Could you check a few things on this model? Use its own coordinates, in mm. Coordinates: 2 decimals unless noted, no trailing zeros. Order: outer loops, then holes, each group sorted by start corner. A loop starts at its lowest first (then second) coordinate and runs counter-clockwise, first axis right, second up. Notation, with made-up numbers: M 17.25,46.5 L 51.25,46.5 A29 ccw 51.25,84.5 Z; hole C -22.75,21 d6. An arc over 180 degrees is marked long. Write item = value, one per line. Start each with the question number.
from build123d import *

# Parameters (mm, degrees)
SKETCH2_R           = 1.75
BOSS_EXTRUDE1_DEPTH = 1
BOSS_EXTRUDE3_START = -1
SKETCH4_R           = 1.75
SKETCH4_R_2         = 1.744098306
BOSS_EXTRUDE3_DEPTH = 1


with BuildPart() as part:
    # Sketch2 → Boss-Extrude1 (new body)
    with BuildSketch(Plane.XY):
        with BuildLine():
            Line((0, 3), (0, 27))
            ThreePointArc((0, 27), (-0.878679656, 29.121320344), (-3, 30))
            Line((-3, 30), (-97, 30))
            ThreePointArc((-97, 30), (-99.121320344, 29.121320344), (-100, 27))
            Line((-100, 27), (-100, 3))
            ThreePointArc((-100, 3), (-99.121320344, 0.878679656), (-97, 0))
            Line((-97, 0), (-3, 0))
            ThreePointArc((-3, 0), (-0.878679656, 0.878679656), (0, 3))
        make_face()
        with Locations((-96, 18)):
            Circle(SKETCH2_R, mode=Mode.SUBTRACT)
        with Locations((-4, 18)):
            Circle(SKETCH2_R, mode=Mode.SUBTRACT)
        with BuildLine():
            Line((-97, 27), (-3, 27))
            Line((-3, 27), (-3, 21.872983346))
            ThreePointArc((-3, 21.872983346), (-8, 18), (-3, 14.127016654))
            Line((-3, 14.127016654), (-3, 3))
            Line((-3, 3), (-97, 3))
            Line((-97, 3), (-97, 14.127016654))
            ThreePointArc((-97, 14.127016654), (-92, 18), (-97, 21.872983346))
            Line((-97, 21.872983346), (-97, 27))
        make_face(mode=Mode.SUBTRACT)
    extrude(amount=BOSS_EXTRUDE1_DEPTH)

    # Sketch4 → Boss-Extrude3 (add)
    with BuildSketch(Plane.XY.offset(1).offset(BOSS_EXTRUDE3_START)):
        with BuildLine():
            Line((-97.171540794, 30.25), (-2.828459206, 30.25))
            ThreePointArc((-2.828459206, 30.25), (-0.651659826, 29.348340174), (0.25, 27.171540794))
            Line((0.25, 27.171540794), (0.25, 2.828459206))
            ThreePointArc((0.25, 2.828459206), (-0.651659826, 0.651659826), (-2.828459206, -0.25))
            Line((-2.828459206, -0.25), (-97.171540794, -0.25))
            ThreePointArc((-97.171540794, -0.25), (-99.348340174, 0.651659826), (-100.25, 2.828459206))
            Line((-100.25, 2.828459206), (-100.25, 27.171540794))
            ThreePointArc((-100.25, 27.171540794), (-99.348340174, 29.348340174), (-97.171540794, 30.25))
        make_face()
        with Locations((-96, 18)):
            Circle(SKETCH4_R, mode=Mode.SUBTRACT)
        with Locations((-4, 18)):
            Circle(SKETCH4_R_2, mode=Mode.SUBTRACT)
        with BuildLine():
            Line((-96.75, 26.75), (-3.25, 26.75))
            Line((-3.25, 26.75), (-3.25, 22.183300133))
            ThreePointArc((-3.25, 22.183300133), (-8.25, 18), (-3.25, 13.816699867))
            Line((-3.25, 13.816699867), (-3.25, 3.25))
            Line((-3.25, 3.25), (-96.75, 3.25))
            Line((-96.75, 3.25), (-96.75, 13.816699867))
            ThreePointArc((-96.75, 13.816699867), (-91.75, 18), (-96.75, 22.183300133))
            Line((-96.75, 22.183300133), (-96.75, 26.75))
        make_face(mode=Mode.SUBTRACT)
    extrude(amount=BOSS_EXTRUDE3_DEPTH)


solid = part.part
(1) Imagine slicing it at B-B on y = 18. List the corners of the cut face in (x, z) for me, plus the area to 3 significant figures.
(2) Imagine slicing it at A-A on y = 24. List the corners of the cut face in (x, z) for me, plus the area to 3 significant figures.
(3) Thinking about a two-plate mould opening in Y: for faces 1 (the flat face through (-50, 27, 1)), 2 (the cylindrical face through (-91.75, 17.9, 0.49)), 3 (the cylindrical face through (-0.628, 0.676, 0.493)), which applies, released by +Y, released by -Y, zero draft, split by the parting line, or undercut?
(4) Please list where these lines run through material, in increasing order: probe 1 along Y at (x, z) = (-96, 0.5); probe 2 along Y at (x, z) = (-83.5, 0.15); probe 3 along Y at (x, z) = (-7.5, 0.65). Write a range as from..to.
(5) Imagine slicing it at D-D on z = 0.25. List the corners of the cut face in (x, y) for me.
(6) Imagine slicing it at C-C on x = -51.5. List the corners of the cut face in (y, z) for me, plus the area to 3 significant figures.
Response:
q1.outline = M -100.25,0 L -97.75,0 L -97.75,1 L -100.25,1 Z; M -94.25,0 L -91.75,0 L -91.75,1 L -94.25,1 Z; M -8.25,0 L -5.74,0 L -5.74,1 L -8.25,1 Z; M -2.26,0 L 0.25,0 L 0.25,1 L -2.26,1 Z
q1.area = 10.0 mm2
q2.outline = M -100.25,0 L -96.75,0 L -96.75,1 L -100.25,1 Z; M -3.25,0 L 0.25,0 L 0.25,1 L -3.25,1 Z
q2.area = 7.00 mm2
q3.face_1 = zero draft
q3.face_2 = undercut
q3.face_3 = released by -Y
q4.probe_1 = -0.25..3.25, 13.75..16.25, 19.75..22.25, 26.75..30.25
q4.probe_2 = -0.25..3.25, 26.75..30.25
q4.probe_3 = -0.25..3.25, 15.59..20.41, 26.75..30.25
q5.outline = M -100.25,2.83 A3.08 ccw -97.17,-0.25 L -2.83,-0.25 A3.08 ccw 0.25,2.83 L 0.25,27.17 A3.08 ccw -2.83,30.25 L -97.17,30.25 A3.08 ccw -100.25,27.17 Z; hole C -96,18 d3.5; hole M -96.75,3.25 L -3.25,3.25 L -3.25,13.82 A4.25 cw long -3.25,22.18 L -3.25,26.75 L -96.75,26.75 L -96.75,22.18 A4.25 cw long -96.75,13.82 Z; hole C -4,18 d3.49
q6.outline = M -0.25,0 L 3.25,0 L 3.25,1 L -0.25,1 Z; M 26.75,0 L 30.25,0 L 30.25,1 L 26.75,1 Z
q6.area = 7.00 mm2
